CAD build for the part. Positions are in the model's coordinates, mm. Give positions to 0.01 mm unless a question says otherwise; leave off trailing zeros. Write each loop counter-clockwise with the first axis right and the second up, starting at its lowest first coordinate (ties: lowest second). Pieces come first, ordered by that corner, then holes. Notation, with made-up numbers: (-35.75, -15.75) -> (23.25, -15.75) arc R18 cw to (23.25, 13.25) -> close; hole circle Ø4 at (-0.75, -12.75). An arc over 180 degrees is marked (long way). Answer in a Markdown table with one row per item. Add a question column.
Autodesk Inventor part; units mm, degrees
ref_plane "우측면도" through (0, 0, 0) normal (1, 0, 0) x (0, 1, 0)
ref_plane "평면도" through (0, 0, 0) normal (0, 1, 0) x (-1, 0, 0)
ref_plane "정면도" through (0, 0, 0) normal (0, 0, 1) x (1, 0, 0)
sketch "스케치1" plane through (0, 0, 0) normal (0, 0, 1) x (1, 0, 0)
  line L0 (0, 0) -> (100, 0)
  line L1 (100, 0) -> (100, 33)
  line L2 (100, 33) -> (0, 33)
  line L3 (0, 33) -> (0, 0)
  dimension "d0" = 100
  dimension "d1" = 33
extrude "돌출1" add sketch "스케치1" along normal blind 3
fillet "모깎기1" radius 3 4 edges at (0, 33, 1.5) (0, 0, 1.5) (100, 0, 1.5) (100, 33, 1.5)
sketch "스케치2" plane through (0, 0, 3) normal (0, 0, 1) x (1, 0, 0)
  circle A0 centre (3, 30) radius 1.5
  circle A1 centre (3, 30) radius 3
  line L0 (100, 33) -> (0, 33)
  line L1 (0, 33) -> (0, 0)
  circle A2 centre (97, 30) radius 1.5
  circle A3 centre (97, 30) radius 3
  circle A4 centre (3, 3) radius 1.5
  circle A5 centre (3, 3) radius 3
  circle A6 centre (97, 3) radius 1.5
  circle A7 centre (97, 3) radius 3
  dimension "d4" = 3
  dimension "d5" = 6
  dimension "d8" = 94
  dimension "d11" = 27
extrude "돌출2" cut sketch "스케치2" against normal blind 4 contours A0 | A2 | A4 | A6
sketch "스케치3" plane through (0, 0, 3) normal (0, 0, 1) x (1, 0, 0)
  line L0 (45, 31.5) -> (75, 31.5) construction
  line L1 (75, 31.5) -> (75, 1.5) construction
  line L2 (75, 1.5) -> (45, 1.5) construction
  line L3 (45, 1.5) -> (45, 31.5) construction
  line L4 (100, 3) -> (100, 30)
  line L5 (3, 0) -> (97, 0)
  line L6 (97, 33) -> (3, 33)
  circle A0 centre (60, 16.5) radius 15
  point P0 (0, 0)
  dimension "d28" = 25
  dimension "d29" = 1.5
  dimension "d30" = 1.5
  dimension "d33" = 30
extrude "돌출3" cut sketch "스케치3" against normal blind 4
equation "\"d8\" = d0 - d5"
equation "\"d11\" = d1 - d5"
equation "\"d30\" = d29"
properties part number "덮개"
Item 1: Slice it at A-A, the plane y = 16.5. List the corners of the cut face in (x, z), then the cut area to 3 significant figures.
Item 2: Mould opens along X. For faces 1 (the face through (97.69, 1.67, 1.52)), 2 (the face through (38, 17, 0)), 3 (the face through (0.9, 32.14, 1.52)) say: released by +X, released by -X, zero draft, split by the parting line, or undercut.
Item 3: Drop a flat-ended pin along its axis: pin 1 Ø2.5 at (x, y) = (3, 3) entering from +Z. Give the stop position or say it passes through.
Item 4: Slice it at B-B, the plane x = 60. List the corners of the cut face in (y, z).
Item 5: Probe L1, parallel to Y at x = 3, z = 1.15; L2, parallel to Y at x = 51, z = 1.8; L3, parallel to X at y = 29, z = 2.85. List the from-to ranges inside material, lowest first. Write a range as from..to.
Item 6: Slice it at C-C, the plane z = 1.8. List the corners of the cut face in (x, y), then the cut area to 3 significant figures.
Answer key:
| question | item | result |
|---|---|---|
| 1 | outline | (0, 0) -> (45, 0) -> (45, 3) -> (0, 3) -> close; (75, 0) -> (100, 0) -> (100, 3) -> (75, 3) -> close |
| 1 | area | 210 mm² |
| 2 | face 1 | undercut |
| 2 | face 2 | zero draft |
| 2 | face 3 | released by -X |
| 3 | pin 1 | passes through |
| 4 | outline | (0, 0) -> (1.5, 0) -> (1.5, 3) -> (0, 3) -> close; (31.5, 0) -> (33, 0) -> (33, 3) -> (31.5, 3) -> close |
| 5 | L1 | y = 0..1.5, 4.5..28.5, 31.5..33 |
| 5 | L2 | y = 0..4.5, 28.5..33 |
| 5 | L3 | x = 0..1.88, 4.12..51.71, 68.29..95.88, 98.12..100 |
| 6 | outline | (0, 3) arc R3 ccw to (3, 0) -> (97, 0) arc R3 ccw to (100, 3) -> (100, 30) arc R3 ccw to (97, 33) -> (3, 33) arc R3 ccw to (0, 30) -> close; hole circle Ø3 at (3, 3); hole circle Ø3 at (3, 30); hole circle Ø30 at (60, 16.5); hole circle Ø3 at (97, 3); hole circle Ø3 at (97, 30) |
| 6 | area | 2,560 mm² |
